```python
from build123d import *

# Parameters (mm, degrees)
CHAMFER1_SIZE = 0.08


with BuildPart() as part:
    # Sketch1 → Revolve1 (revolve)
    with BuildSketch(Plane.XY):
        with BuildLine():
            Line((-1.6, -4), (-0.9367497, -4))
            ThreePointArc((-0.9367497, -4), (0, -4.45), (0.9367497, -4))
            Line((0.9367497, -4), (1.6, -4))
            Line((1.6, -4), (1.6, -4.1))
            Line((1.6, -4.1), (1.8, -4.1))
            Line((1.8, -4.1), (1.8, -4))
            Line((1.8, -4), (2, -4))
            Line((2, -4), (2, -5))
            Line((2, -5), (-2, -5))
            Line((-2, -5), (-2, -4))
            Line((-2, -4), (-1.8, -4))
            Line((-1.8, -4), (-1.8, -4.1))
            Line((-1.8, -4.1), (-1.6, -4.1))
            Line((-1.6, -4.1), (-1.6, -4))
        make_face()
    revolve(axis=Axis((-6.429017492, 0, 0), (1, 0, 0)))

    # Chamfer1
    chamfer1_edges = [part.edges().sort_by_distance(p)[0] for p in [
        (2, 5, 0),
        (-2, 5, 0),
        (-2, 4, 0),
        (2, 4, 0),
    ]]
    chamfer(chamfer1_edges, length=CHAMFER1_SIZE)


solid = part.part
```
For this review, take the finished solid that the model builds, in its own axes (mm). Coordinates: 2 decimals unless noted, no trailing zeros. Write each loop counter-clockwise with the first axis right and the second up, starting at its lowest first coordinate (ties: lowest second). Pieces come first, ordered by that corner, then holes. Notation, with made-up numbers: (83.25, 40.25) - (118.25, 40.25) arc R13 cw to (118.25, 59.25) - close; hole circle Ø4 at (23, 51). An arc over 180 degrees is marked (long way). Put each result on its own line as item: value.
1. Add section A-A, the plane x = -0.65. Give the boundary of the cut face in (y, z), then the cut area to 3 significant figures.
Values found:
outline: circle Ø10 at (0, 0); hole circle Ø8.52 at (0, 0)
area: 21.6 mm²
2. Mouldability with a two-part tool opening along Z and no side actions: class faces 1 (the cylindrical face through (-1.264, 0.867, 3.905)), 2 (the flat face through (2, -2, -4)), 3 (the cylindrical face through (1.273, 0.867, 3.905)), 4 (the cylindrical face through (-0.03, 1.08, 4.88)) as released by +Z, released by -Z, zero draft, split by the parting line, or undercut.
Values found:
face 1: undercut
face 2: zero draft
face 3: undercut
face 4: split by the parting line
3. For pin 1 (1.5 mm diameter, centred on x = -0.5, y = 2, fed in from -Z); pin 2 (4 mm diameter, centred on y = 1, z = -1.5, fed in from +X), all flat-tipped, find the tip position at first contact; note any pin that passes through.
Values found:
pin 1: z = -4.84
pin 2: through
4. Wall thickness on probe 1 along Y at (x, z) = (-1.35, 0); probe 2 along Y at (x, z) = (-1.7, 0): over which ranges is each line inside the solid? List them lowest first.
Values found:
probe 1: -5 to -4, 4 to 5
probe 2: -5 to -4.1, 4.1 to 5
5. Add section B-B, the plane x = 0.4. Give the boundary of the cut face in (y, z), then the cut area to 3 significant figures.
Values found:
outline: circle Ø10 at (0, 0); hole circle Ø8.76 at (0, 0)
area: 18.2 mm²
